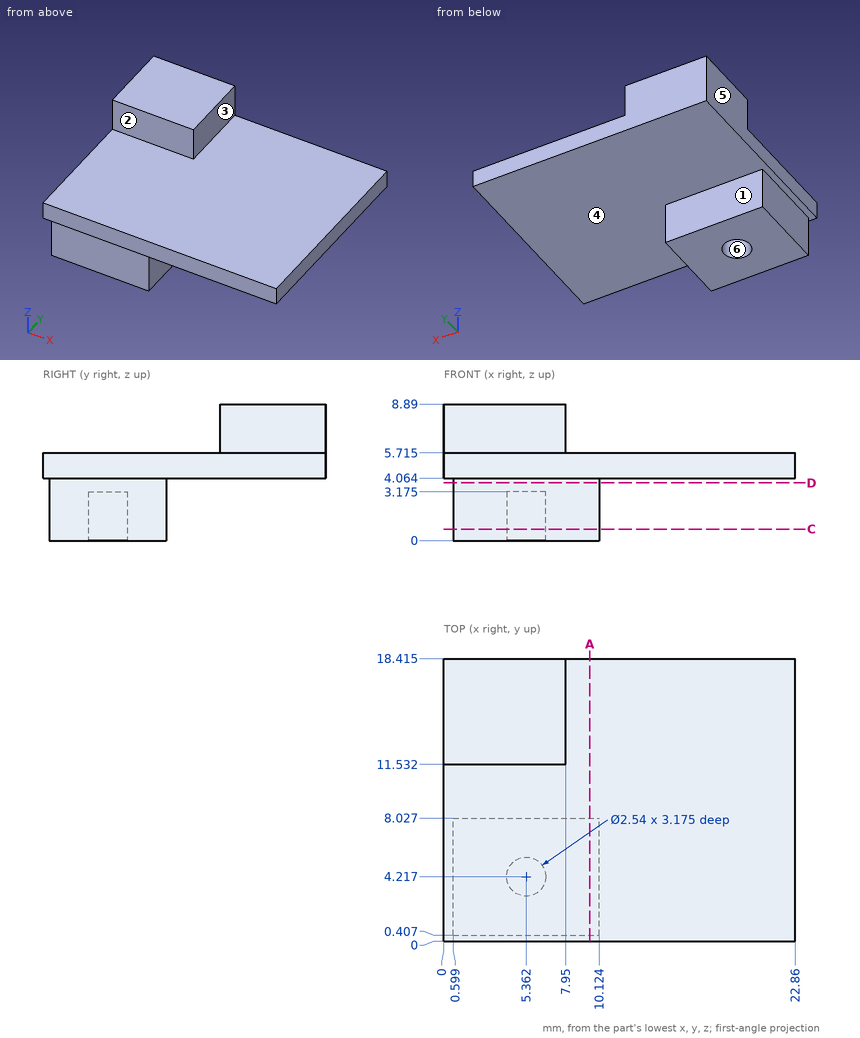
Design review of the part shown in the three views and the two pictorial views. Dimensions are in mm from the part's minimum x, y and z. A direction names the side the tool comes from. Round coordinates to 2 decimals unless told otherwise and drop trailing zeros. Order: outer loops, then holes, each group sorted by start corner. A loop starts at its lowest first (then second) coordinate and runs counter-clockwise, first axis right, second up. Notation, with made-up numbers: (39, 39.5) - (59, 39.5) arc R11 ccw to (59, 50.5) - close; hole circle Ø4 at (-11.5, 64). An arc over 180 degrees is marked (long way). Answer in a Markdown table with one row per item.
(1) Clearance check with flat-ended pins moving along their axes: P1, Ø1.2, axis at y = 3, z = 2, coming from the +X side (1 decimal); P2, Ø3.5, axis at y = 3.5, z = 1, coming from the -X side; P3, Ø8, axis at x = 17.5, y = 16, coming from the -Z side. State where each tip first meets the part, or that it passes through.
Result set:
| item | result |
|---|---|
| P1 | stops at x = 10.1 |
| P2 | stops at x = 0.6 |
| P3 | stops at z = 4.06 |
(2) Take a section at C-C on z = 0.75. Write out the cut boundary in (x, y) (1 decimal).
Result set:
| item | result |
|---|---|
| outline | (0.6, 0.4) - (10.1, 0.4) - (10.1, 8) - (0.6, 8) - close; hole circle Ø2.5 at (5.4, 4.2) |
(3) Take a section at D-D on z = 3.75. Write out the cut boundary in (x, y) (1 decimal).
Result set:
| item | result |
|---|---|
| outline | (0.6, 0.4) - (10.1, 0.4) - (10.1, 8) - (0.6, 8) - close |
(4) For line 1 (Z direction, x = 3.25, y = 7.5) (1 decimal); line 2 (X direction, y = 6, z = 3) (1 decimal); line 3 (Z direction, x = 12.25, y = 4) (1 decimal), list the stretches that pass through material, from the lowest coordinate up. Write a range as from..to.
Result set:
| item | result |
|---|---|
| line 1 | z = 0..5.7 |
| line 2 | x = 0.6..10.1 |
| line 3 | z = 4.1..5.7 |
(5) Mouldability with a two-part tool opening along X and no side actions: class the marked faces 4, 5 and 6 as released by +X, released by -X, zero draft, split by the parting line, or undercut.
Result set:
| item | result |
|---|---|
| face 4 | zero draft |
| face 5 | released by -X |
| face 6 | undercut |
(6) Machinability: for the marked faces 1, 2 and 3, which of the approach directions +Z, -Z, +X, -X, +Y, -Y give a long, thin tool a straight path to every point of the face, cutting with its end or side? Answer none if there is none.
Result set:
| item | result |
|---|---|
| face 1 | -Z, +X, -X, +Y |
| face 2 | +Z, +X, -X, -Y |
| face 3 | +Z, +X, +Y, -Y |
(7) Take a section at A-A on x = 9.5. Write out the cut boundary in (y, z) (1 decimal).
Result set:
| item | result |
|---|---|
| outline | (0, 4.1) - (0.4, 4.1) - (0.4, 0) - (8, 0) - (8, 4.1) - (18.4, 4.1) - (18.4, 5.7) - (0, 5.7) - close |
